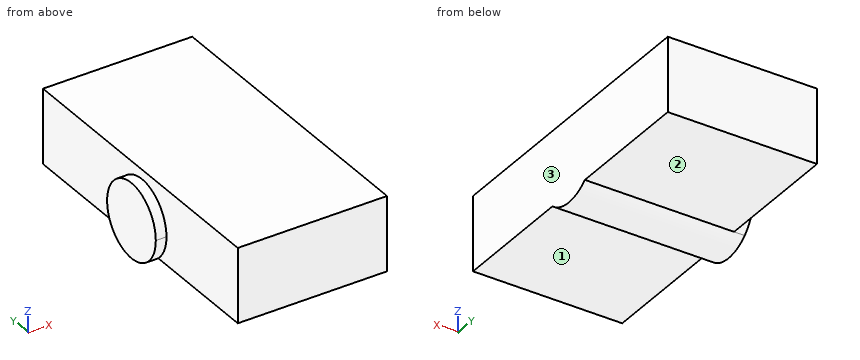
```python
from build123d import *

# Parameters (mm, degrees)
F0_W          = 355.6
F0_H          = 711.2
F1_DEPTH      = 177.8
F3_DEPTH      = 25.4
F3_DEPTH_BACK = 355.6


with BuildPart() as f1:
    # F0 (on Top) → F1 (new body)
    with BuildSketch(Plane.XY):
        with Locations((-177.8, 355.6)):
            Rectangle(F0_W, F0_H)
    extrude(amount=-F1_DEPTH)

    # F2 (on face) → F3 (join, two sides)
    with BuildSketch(Plane(origin=(-355.6, 0, 0), x_dir=(0, -1, 0), z_dir=(-1, 0, 0))) as f3_sk:
        with BuildLine():
            ThreePointArc((-290.325146, -177.8), (-268.245349, -147.75703), (-260.427027, -111.30197))
            ThreePointArc((-260.427027, -111.30197), (-385.782087, -30.220291), (-408.328908, -177.8))
            Line((-408.328908, -177.8), (-290.325146, -177.8))
        make_face()
        with BuildLine():
            Line((-290.325146, -177.8), (-408.328908, -177.8))
            ThreePointArc((-408.328908, -177.8), (-349.327027, -200.20197), (-290.325146, -177.8))
        make_face()
    extrude(amount=F3_DEPTH)
    extrude(f3_sk.sketch, amount=-F3_DEPTH_BACK)


solid = f1.part
```
Work out the finished part from the listing and answer in its coordinate system (mm). Face numbers are marked on the shaded views. A direction names the side the tool comes from. Coordinates: 2 decimals unless noted, no trailing zeros. Write each loop counter-clockwise with the first axis right and the second up, starting at its lowest first coordinate (ties: lowest second). Pieces come first, ordered by that corner, then holes. Notation, with made-up numbers: (41.5, 43.5) - (87.5, 43.5) arc R25 ccw to (87.5, 78.5) - close; hole circle Ø1 at (2, -19). An arc over 180 degrees is marked (long way). Answer as a JSON object with one key per item and string values.
Q1. Find section C-C (y = 430). Write down the section's boundary in (x, z), plus the area to 3 significant figures.
Results list:
{"outline": "(-381, -148.65) - (-355.6, -148.65) - (-355.6, -177.8) - (0, -177.8) - (0, 0) - (-355.6, 0) - (-355.6, -73.95) - (-381, -73.95) - close", "area": "65,100 mm^2"}
Q2. Given pin 1 Ø3 at (x, y) = (-119.5, 369.5) entering from -Z, flat-ended and moving along its own axis, determine where the tip first touches the part or whether it passes through.
Results list:
{"pin 1": "stops at z = -198.22"}
Q3. Find section A-A (x = -167). Write down the section's boundary in (y, z).
Results list:
{"outline": "(0, -177.8) - (290.33, -177.8) arc R88.9 ccw to (408.33, -177.8) - (711.2, -177.8) - (711.2, 0) - (0, 0) - close"}
Q4. Which of the six approach directions +Z, -Z, +X, -X, +Y, -Y give full straight-line access (tool end or side, diameter ignored) to the marked faces 1, 2 and 3?
Results list:
{"face 1": "-Z, +X, -X, -Y", "face 2": "-Z, +X, -X, +Y", "face 3": "+Z, -Z, +X, +Y, -Y"}
Q5. Find section D-D (y = 612.5). Write down the section's boundary in (x, z).
Results list:
{"outline": "(-355.6, -177.8) - (0, -177.8) - (0, 0) - (-355.6, 0) - close"}
Q6. Consider L1, parallel to X at y = 109.5, z = -78; L2, parallel to Z at x = -30, y = 184.5; L3, parallel to Z at x = -23, y = 351. Determine where each line is inside the solid, lowest interval first. Write a range as from..to.
Results list:
{"L1": "x = -355.6..0", "L2": "z = -177.8..0", "L3": "z = -200.19..0"}
Q7. Find section B-B (z = -30). Write down the section's boundary in (x, y).
Results list:
{"outline": "(-381, 313.37) - (-355.6, 313.37) - (-355.6, 0) - (0, 0) - (0, 711.2) - (-355.6, 711.2) - (-355.6, 385.29) - (-381, 385.29) - close"}
